Build history of the part. All positions in model axes, mm. A direction names the side the tool comes from. Give positions to 0.01 mm unless a question says otherwise; leave off trailing zeros. Use a Markdown table: item, result.
from build123d import *

# Parameters (mm, degrees)
EXTRUDE_1_DEPTH             = 38
SKETCH_3_R                  = 4.35
EXTRUDE_2_DEPTH             = 838
EXTRUDE_3_DEPTH             = 38
SKETCH_5_W                  = 42
SKETCH_5_H                  = 22.5
PATTERN_LINEAR_1_COUNT      = 2
PATTERN_LINEAR_1_PITCH      = 72
PATTERN_LINEAR_1_COUNT_DIR2 = 2
PATTERN_LINEAR_1_PITCH_DIR2 = 72
PATTERN_LINEAR_2_COUNT      = 2
PATTERN_LINEAR_2_PITCH      = 72
PATTERN_LINEAR_2_COUNT_DIR2 = 2
PATTERN_LINEAR_2_PITCH_DIR2 = 72


with BuildPart() as part:
    # Sketch 1 → Extrude 1 (new body)
    with BuildSketch(Plane(origin=(0, 0, 0), x_dir=(0, 0, -1), z_dir=(1, 0, 0))):
        with BuildLine():
            Line((-43.5, -47.5), (43.5, -47.5))
            ThreePointArc((43.5, -47.5), (46.328427125, -46.328427125), (47.5, -43.5))
            Line((47.5, -43.5), (47.5, 43.5))
            ThreePointArc((47.5, 43.5), (46.328427125, 46.328427125), (43.5, 47.5))
            Line((43.5, 47.5), (-43.5, 47.5))
            ThreePointArc((-43.5, 47.5), (-46.328427125, 46.328427125), (-47.5, 43.5))
            Line((-47.5, 43.5), (-47.5, -43.5))
            ThreePointArc((-47.5, -43.5), (-46.328427125, -46.328427125), (-43.5, -47.5))
        make_face()
    extrude(amount=EXTRUDE_1_DEPTH)

    # Sketch 2 → Revolve 1 (revolve)
    with BuildSketch(Plane(origin=(0, 0, 0), x_dir=(1, 0, 0), z_dir=(0, 1, 0))):
        with BuildLine():
            Line((-20, 0), (-20, 19))
            ThreePointArc((-20, 19), (-19.707106781, 19.707106781), (-19, 20))
            Line((-19, 20), (-5, 20))
            Line((-5, 20), (-5, 21.5))
            ThreePointArc((-5, 21.5), (-4.707106781, 22.207106781), (-4, 22.5))
            Line((-4, 22.5), (38, 22.5))
            Line((38, 22.5), (38, 0))
            Line((38, 0), (-20, 0))
        make_face()
    revolve(axis=Axis((38, 0, 0), (-1, 0, 0)))

    # Sketch 3 → Extrude 2 (add)
    with BuildSketch(Plane(origin=(38, 0, 0), x_dir=(0, 0, -1), z_dir=(1, 0, 0))):
        with BuildLine():
            Line((-31.780252532, -41.679747468), (-26.587928413, -36.48742335))
            ThreePointArc((-26.587928413, -36.48742335), (-25.372501394, -35.911540455), (-24.067177934, -36.235630894))
            ThreePointArc((-24.067177934, -36.235630894), (0, -43.5), (24.067177934, -36.235630894))
            ThreePointArc((24.067177934, -36.235630894), (25.372501394, -35.911540455), (26.587928413, -36.48742335))
            Line((26.587928413, -36.48742335), (31.780252532, -41.679747468))
            ThreePointArc((31.780252532, -41.679747468), (41.679747468, -41.679747468), (41.679747468, -31.780252532))
            Line((41.679747468, -31.780252532), (36.48742335, -26.587928413))
            ThreePointArc((36.48742335, -26.587928413), (35.911540455, -25.372501394), (36.235630894, -24.067177934))
            ThreePointArc((36.235630894, -24.067177934), (43.5, 0), (36.235630894, 24.067177934))
            ThreePointArc((36.235630894, 24.067177934), (35.911540455, 25.372501394), (36.48742335, 26.587928413))
            Line((36.48742335, 26.587928413), (41.679747468, 31.780252532))
            ThreePointArc((41.679747468, 31.780252532), (41.679747468, 41.679747468), (31.780252532, 41.679747468))
            Line((31.780252532, 41.679747468), (26.587928413, 36.48742335))
            ThreePointArc((26.587928413, 36.48742335), (25.372501394, 35.911540455), (24.067177934, 36.235630894))
            ThreePointArc((24.067177934, 36.235630894), (0, 43.5), (-24.067177934, 36.235630894))
            ThreePointArc((-24.067177934, 36.235630894), (-25.372501394, 35.911540455), (-26.587928413, 36.48742335))
            Line((-26.587928413, 36.48742335), (-31.780252532, 41.679747468))
            ThreePointArc((-31.780252532, 41.679747468), (-41.679747384, 41.679747384), (-41.679747468, 31.780252532))
            Line((-41.679747468, 31.780252532), (-36.48742335, 26.587928413))
            ThreePointArc((-36.48742335, 26.587928413), (-35.911540455, 25.372501394), (-36.235630894, 24.067177934))
            ThreePointArc((-36.235630894, 24.067177934), (-43.5, 0), (-36.235630894, -24.067177934))
            ThreePointArc((-36.235630894, -24.067177934), (-35.911540455, -25.372501394), (-36.48742335, -26.587928413))
            Line((-36.48742335, -26.587928413), (-41.679747468, -31.780252532))
            ThreePointArc((-41.679747468, -31.780252532), (-41.679747384, -41.679747384), (-31.780252532, -41.679747468))
        make_face()
        with Locations((36, 36)):
            Circle(SKETCH_3_R, mode=Mode.SUBTRACT)
        with Locations((36, -36)):
            Circle(SKETCH_3_R, mode=Mode.SUBTRACT)
        with Locations((-36, 36)):
            Circle(SKETCH_3_R, mode=Mode.SUBTRACT)
        with Locations((-36, -36)):
            Circle(SKETCH_3_R, mode=Mode.SUBTRACT)
    extrude(amount=EXTRUDE_2_DEPTH)

    # Sketch 4 → Extrude 3 (add)
    with BuildSketch(Plane(origin=(914, 0, 0), x_dir=(0, 0, -1), z_dir=(1, 0, 0))):
        with BuildLine():
            Line((-43.5, -47.5), (43.5, -47.5))
            ThreePointArc((43.5, -47.5), (46.328427125, -46.328427125), (47.5, -43.5))
            Line((47.5, -43.5), (47.5, 43.5))
            ThreePointArc((47.5, 43.5), (46.328427125, 46.328427125), (43.5, 47.5))
            Line((43.5, 47.5), (-43.5, 47.5))
            ThreePointArc((-43.5, 47.5), (-46.328427125, 46.328427125), (-47.5, 43.5))
            Line((-47.5, 43.5), (-47.5, -43.5))
            ThreePointArc((-47.5, -43.5), (-46.328427125, -46.328427125), (-43.5, -47.5))
        make_face()
    extrude(amount=-EXTRUDE_3_DEPTH)

    # Sketch 5 → Revolve 2 (revolve)
    with BuildSketch(Plane.XY):
        with Locations((897, 11.25)):
            Rectangle(SKETCH_5_W, SKETCH_5_H)
    revolve(axis=Axis((918, 0, 0), (-1, 0, 0)))

    # Sketch 6 → Cut-Revolve 1 (revolve, cut)
    with BuildSketch(Plane(origin=(0, 11.5, 0), x_dir=(1, 0, 0), z_dir=(0, 1, 0))):
        Polygon((19, -47.5), (10.669, -47.5), (11.525, -46.644), (11.525, -29.5), (19, -25.184306738), align=None)
    revolve(axis=Axis((19, 11.5, 25.184306738), (0, 0, 1)), mode=Mode.SUBTRACT)

    # Sketch 7 → Cut-Revolve 2 (revolve, cut)
    with BuildSketch(Plane(origin=(0, 11.5, 0), x_dir=(1, 0, 0), z_dir=(0, 1, 0))):
        Polygon((895, -47.5), (886.669, -47.5), (887.525, -46.644), (887.525, -29.5), (895, -25.184306738), align=None)
    revolve(axis=Axis((895, 11.5, 25.184306738), (0, 0, 1)), mode=Mode.SUBTRACT)

    # Sketch 8 → Cut-Revolve 3 (revolve, cut)
    with BuildSketch(Plane(origin=(0, -14, 0), x_dir=(1, 0, 0), z_dir=(0, 1, 0))):
        Polygon((26.5, -47.5), (20.95, -47.5), (21.45, -47), (21.45, -44), (21.95, -44), (21.95, -46.5), (22.45, -47), (24, -47), (24, -44), (26.5, -44), align=None)
    revolve(axis=Axis((26.5, -14, 44), (0, 0, 1)), mode=Mode.SUBTRACT)

    # Sketch 9 → Cut-Revolve 4 (revolve, cut)
    with BuildSketch(Plane(origin=(0, -14, 0), x_dir=(1, 0, 0), z_dir=(0, 1, 0))):
        Polygon((887.5, -47.5), (881.95, -47.5), (882.45, -47), (882.45, -44), (882.95, -44), (882.95, -46.5), (883.45, -47), (885, -47), (885, -44), (887.5, -44), align=None)
    revolve(axis=Axis((887.5, -14, 44), (0, 0, 1)), mode=Mode.SUBTRACT)

    # Sketch 10 → Cut-Revolve 5 (revolve, cut)
    with BuildSketch(Plane.XY.offset(-36)):
        Polygon((20, -36), (20, -40.188), (8.812, -40.188), (8, -41), (8, -43.95), (0, -43.95), (0, -36), align=None)
    cut_revolve_5 = revolve(axis=Axis((0, -36, -36), (1, 0, 0)), mode=Mode.SUBTRACT)

    # Pattern Linear 1: Cut-Revolve 5 2 × 2
    with Locations(*[(0, i * PATTERN_LINEAR_1_PITCH, j * PATTERN_LINEAR_1_PITCH_DIR2) for i in range(PATTERN_LINEAR_1_COUNT) for j in range(PATTERN_LINEAR_1_COUNT_DIR2) if (i, j) != (0, 0)]):
        add(cut_revolve_5, mode=Mode.SUBTRACT)

    # Sketch 12 → Cut-Revolve 6 (revolve, cut)
    with BuildSketch(Plane.XY.offset(-36)):
        Polygon((914, -36), (914, -43.95), (906, -43.95), (906, -41), (905.188, -40.188), (894, -40.188), (894, -36), align=None)
    cut_revolve_6 = revolve(axis=Axis((894, -36, -36), (1, 0, 0)), mode=Mode.SUBTRACT)

    # Pattern Linear 2: Cut-Revolve 6 2 × 2
    with Locations(*[(0, i * PATTERN_LINEAR_2_PITCH, j * PATTERN_LINEAR_2_PITCH_DIR2) for i in range(PATTERN_LINEAR_2_COUNT) for j in range(PATTERN_LINEAR_2_COUNT_DIR2) if (i, j) != (0, 0)]):
        add(cut_revolve_6, mode=Mode.SUBTRACT)

    # Sketch 14 → Cut-Revolve 7 (revolve, cut)
    with BuildSketch(Plane.XY):
        Polygon((-20, 0), (-20, 12.5), (-1.5, 12.5), (-1.5, 18.2), (34.5, 18.2), (34.5, 40), (879.5, 40), (879.5, 18.2), (915.5, 18.2), (915.5, 0), align=None)
    revolve(axis=Axis((915.5, 0, 0), (-1, 0, 0)), mode=Mode.SUBTRACT)


solid = part.part
1) Tool access for faces 1 (the cylindrical face through (3.944, -34.965, 28.118)), 2 (the cylindrical face through (909.944, 37.035, -43.882)), 3 (the flat face through (915.5, 0, 0)), 4 (the flat face through (19, 47.5, -1)): list every direction of +Z, -Z, +X, -X, +Y, -Y with a clear straight run to the whole face (end or side of a thin tool).
Computed:
| item | result |
|---|---|
| face 1 | -X |
| face 2 | +X |
| face 3 | none |
| face 4 | +Z, -Z, +X, -X, +Y |
2) Slice it at A-A (x = 156.5). State how many separate pieces and enclosed holes the cut face has, and give its area (3 significant figures).
Computed:
| item | result |
|---|---|
| separate pieces | 1 |
| enclosed holes | 5 |
| area | 1,480 mm² |
3) Two-plate mould, pull along Z, no slides. Class faces 5 (the cylindrical face through (15.55, 18.13, 37.95)), 6 (the cylindrical face through (451.1, -0.4, -43.5)), 7 (the flat face through (8, 35.9, -30.8)): +Z half, -Z half, draft (parallel to the pull), parting line (faces both ways), or undercut.
Computed:
| item | result |
|---|---|
| face 5 | draft |
| face 6 | -Z half |
| face 7 | undercut |
4) Pin check, flat tips, straight feed: P1, Ø2, axis at x = 379, z = 35, coming from the +Y side; P2, Ø8, axis at x = 444, y = 10, coming from the -Z side; P3, Ø1, axis at x = 460, y = 26.5, coming from the -Z side; P4, Ø24, axis at x = 895, y = 11.5, coming from the +Z side. Stop position of each tip, or through.
Computed:
| item | result |
|---|---|
| P1 | stops at y = 43.69 |
| P2 | stops at z = -43.08 |
| P3 | stops at z = -36.9 |
| P4 | stops at z = 47.5 |
5) Wall check: line 1 (Y direction, x = 53.5, z = -3.5); line 2 (X direction, y = 14, z = -21); line 3 (Y direction, x = 193, z = -24). Give the ranges that are in metal, low to high. Write a range as from..to.
Computed:
| item | result |
|---|---|
| line 1 | y = -43.36..-39.85, 39.85..43.36 |
| line 2 | x = 0..34.5, 879.5..914 |
| line 3 | y = -36.28..-32, 32..36.28 |
